from build123d import *

# Parameters (mm, degrees)
SKETCH2_R           = 1.075
SKETCH2_R_2         = 2.75
BOSS_EXTRUDE1_DEPTH = 5.15
SHELL1_T            = -1.1


with BuildPart() as part:
    # Sketch2 → Boss-Extrude1 (new body)
    with BuildSketch(Plane(origin=(0, 0, 0), x_dir=(1, 0, 0), z_dir=(0, 1, 0))):
        with BuildLine():
            Line((0, 10.1), (20, 10.1))
            Line((20, 10.1), (20, -10.1))
            Line((20, -10.1), (0, -10.1))
            ThreePointArc((0, -10.1), (-10.1, 0), (0, 10.1))
        make_face()
        with Locations((-4.242640687, 4.242640687)):
            Circle(SKETCH2_R, mode=Mode.SUBTRACT)
        with Locations((4.242640687, 4.242640687)):
            Circle(SKETCH2_R, mode=Mode.SUBTRACT)
        with Locations((-4.242640687, -4.242640687)):
            Circle(SKETCH2_R, mode=Mode.SUBTRACT)
        with Locations((4.242640687, -4.242640687)):
            Circle(SKETCH2_R, mode=Mode.SUBTRACT)
        Circle(SKETCH2_R_2, mode=Mode.SUBTRACT)
    extrude(amount=BOSS_EXTRUDE1_DEPTH)

    # Shell1
    shell1_openings = [part.faces().sort_by_distance(p)[0] for p in [
        (20, 2.575, 0),
    ]]
    offset(amount=SHELL1_T, openings=shell1_openings)


solid = part.part
For this review, take the finished solid that the model builds, in its own axes (mm). A direction names the side the tool comes from. Coordinates: 2 decimals unless noted, no trailing zeros. Order: outer loops, then holes, each group sorted by start corner. A loop starts at its lowest first (then second) coordinate and runs counter-clockwise, first axis right, second up. Notation, with made-up numbers: (33, 85) - (70, 85) arc R17 cw to (70, 98) - close; hole circle Ø10 at (24, 66). An arc over 180 degrees is marked (long way). Use one line per item in the form item = value.
Q1. For probe 1 along Y at (x, z) = (17, 4); probe 2 along X at (y, z) = (3.45, 1); probe 3 along Z at (x, y) = (-3.5, 4.9), list the stretches that pass through material, from the lowest coordinate up. Write a range as from..to.
Checked values:
probe_1 = 0..1.1, 4.05..5.15
probe_2 = -10.05..-8.94, -3.72..-2.56, 2.56..3.72
probe_3 = -9.47..-5.02, -3.47..3.47, 5.02..9.47
Q2. For P1, Ø4.5, axis at x = 0, z = 0, coming from the -Y side; P2, Ø1, axis at y = 2, z = -5.5, coming from the -X side; P3, Ø1.5, axis at x = -3, y = 2, coming from the +Z side; P4, Ø1.5, axis at x = -1, y = 2, coming from the +Z side, all flat-tipped, find the tip position at first contact; note any pin that passes through.
Checked values:
P1 = through
P2 = -8.78
P3 = 9.85
P4 = 10.1
Q3. Consider section C-C (x = 7). Give the boundary of the cut face in (y, z).
Checked values:
outline = (0, -10.1) - (5.15, -10.1) - (5.15, 10.1) - (0, 10.1) - close; hole (1.1, -9) - (4.05, -9) - (4.05, 9) - (1.1, 9) - close
Q4. For faces 5 (the cylindrical face through (0.04, 2.55, -3.85)), 6 (the cylindrical face through (3.45, 2.54, -4.97)), 7 (the flat face through (10, 3, 9)), list the 3-axis set-ups (+Z, -Z, +X, -X, +Y, -Y) from which the entire face can be reached by the end or side of a thin tool; tool diameter is ignored.
Checked values:
face_5 = none
face_6 = +Y, -Y
face_7 = +X
Q5. Consider section A-A (z = 0). Give the boundary of the cut face in (x, y).
Checked values:
outline = (-10.1, 0) - (-2.75, 0) - (-2.75, 5.15) - (-10.1, 5.15) - close; (2.75, 0) - (20, 0) - (20, 1.1) - (3.85, 1.1) - (3.85, 4.05) - (20, 4.05) - (20, 5.15) - (2.75, 5.15) - close; hole (-9, 1.1) - (-3.85, 1.1) - (-3.85, 4.05) - (-9, 4.05) - close
Q6. Consider section D-D (z = 3.5). Give the boundary of the cut face in (x, y).
Checked values:
outline = (-9.47, 0) - (-5.02, 0) - (-5.02, 5.15) - (-9.47, 5.15) - close; (-3.47, 0) - (3.47, 0) - (3.47, 5.15) - (-3.47, 5.15) - close; (5.02, 0) - (20, 0) - (20, 1.1) - (6.29, 1.1) - (6.29, 4.05) - (20, 4.05) - (20, 5.15) - (5.02, 5.15) - close; hole (-8.29, 1.1) - (-6.29, 1.1) - (-6.29, 4.05) - (-8.29, 4.05) - close; hole (-2.2, 1.1) - (-1.6, 1.1) - (-1.6, 4.05) - (-2.2, 4.05) - close; hole (1.6, 1.1) - (2.2, 1.1) - (2.2, 4.05) - (1.6, 4.05) - close
Q7. Draft analysis for pull direction X (two halves, no side actions). For faces 1 (the cylindrical face through (-0.596, 2.539, 2.685)), 2 (the cylindrical face through (-10.1, 2.5, 0.2)), 3 (the flat face through (5, 0, 0)), 4 (the cylindrical face through (3.17, 2.54, 4.2)), state which applies: +X half, -X half, draft (parallel to the pull), parting line (faces both ways), or undercut.
Checked values:
face_1 = undercut
face_2 = -X half
face_3 = draft
face_4 = undercut
Q8. Consider section B-B (y = 2.35). Give the boundary of the cut face in (x, z) (3 decimals), then the cut area to 3 significant figures.
Checked values:
outline = (-2.902, -2.53) arc R2.175 ccw (long way) to (-2.53, -2.902) arc R3.85 ccw to (2.53, -2.902) arc R2.175 ccw (long way) to (2.902, -2.53) arc R3.85 ccw to (2.902, 2.53) arc R2.175 ccw (long way) to (2.53, 2.902) arc R3.85 ccw to (-2.53, 2.902) arc R2.175 ccw (long way) to (-2.902, 2.53) arc R3.85 ccw to start; (0, -10.1) - (20, -10.1) - (20, -9) - (0, -9) arc R9 cw to (0, 9) - (20, 9) - (20, 10.1) - (0, 10.1) arc R10.1 ccw to start; hole circle Ø2.15 at (-4.243, -4.243); hole circle Ø2.15 at (-4.243, 4.243); hole circle Ø5.5 at (0, 0); hole circle Ø2.15 at (4.243, -4.243); hole circle Ø2.15 at (4.243, 4.243)
area = 145 mm2
